Input: dimensioned drawing with shaded views. Units: mm. Origin: part minimum x, y, z. A direction names the side the tool comes from. Round coordinates to 2 decimals unless told otherwise and drop trailing zeros. Write each loop counter-clockwise with the first axis right and the second up, starting at its lowest first coordinate (ties: lowest second). Pieces come first, ordered by that corner, then holes. Notation, with made-up numbers: M -32,82.5 L -4,82.5 A9 ccw -4,92.5 Z; hole C 2.25,-34 d10. An arc over 180 degrees is marked long. Answer as CSV lines item,"result". Start each with the question number.
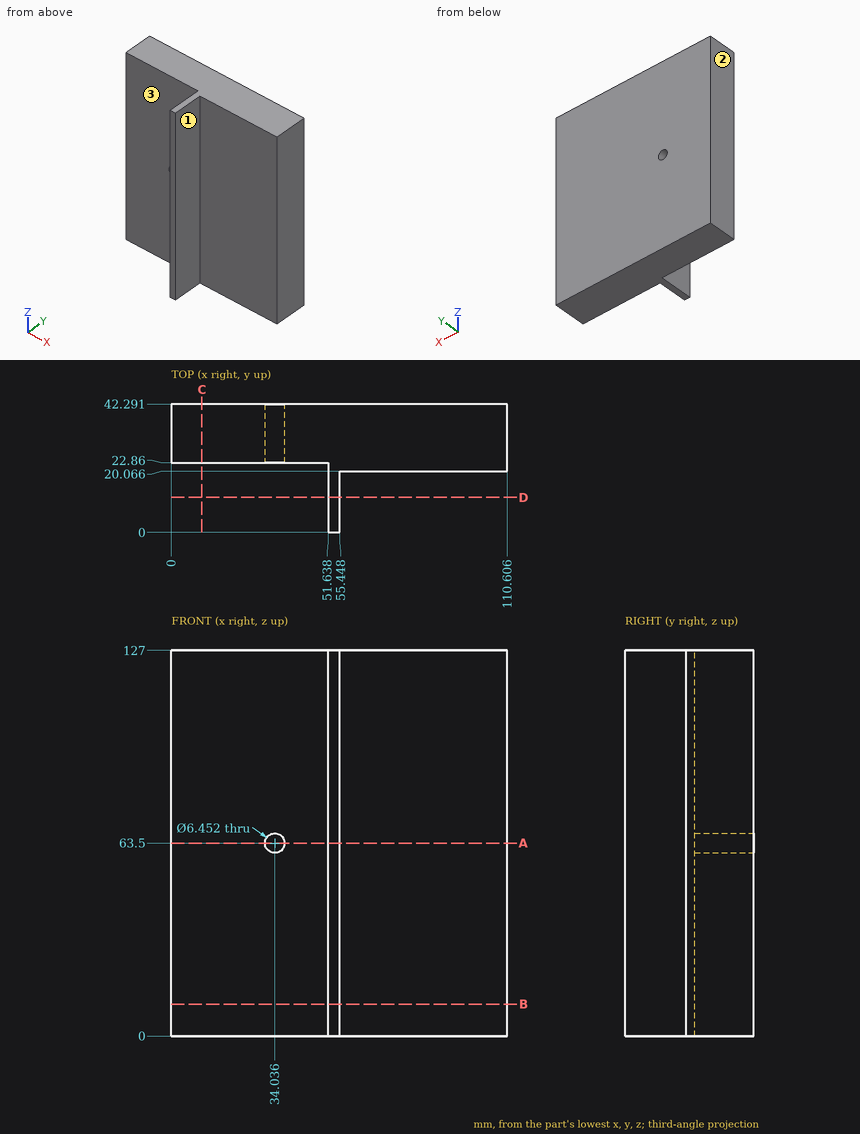
Item 1: Cut plane C-C, the plane x = 10. Return loops of the section in (y, z), plus the area to 3 significant figures.
Item 2: Cut plane D-D, the plane y = 11.5. Return loops of the section in (x, z).
Item 3: Cut plane B-B, the plane z = 10.5. Return loops of the section in (x, y).
Item 4: Cut plane A-A, the plane z = 63.5. Return loops of the section in (x, y), plus the area to 4 significant figures.
Item 5: Pin query (flat end, axial travel): pin 1 Ø1.5 at (x, z) = (22.5, 112) entering from -Y; pin 2 Ø5 at (x, z) = (34.036, 63.5) entering from +Y; pin 3 Ø16.5 at (x, z) = (86.5, 65) entering from -Y. Return the tip coordinate at first contact, or that it passes through.
Item 6: Access query for the marked faces 1, 2 and 3. Directions: +Z, -Z, +X, -X, +Y, -Y. A direction counts if a zero-diameter tool reaches every point of the face in a straight line with its end or side. Return the directions, or none.
Item 7: Line query: line 1 (Y direction, x = 48, z = 102.5); line 2 (X direction, y = 16, z = 29.5); line 3 (Y direction, x = 98, z = 79.5). Output: solid intervals per line, ascending. Write a range as [from, to].
Results list:
1,outline,"M 22.86,0 L 42.29,0 L 42.29,127 L 22.86,127 Z"
1,area,"2,470 mm²"
2,outline,"M 51.64,0 L 55.45,0 L 55.45,127 L 51.64,127 Z"
3,outline,"M 0,22.86 L 51.64,22.86 L 51.64,0 L 55.45,0 L 55.45,20.07 L 110.61,20.07 L 110.61,42.29 L 0,42.29 Z"
4,outline,"M 0,22.86 L 30.81,22.86 L 30.81,42.29 L 0,42.29 Z; M 37.26,22.86 L 51.64,22.86 L 51.64,0 L 55.45,0 L 55.45,20.07 L 110.61,20.07 L 110.61,42.29 L 37.26,42.29 Z"
4,area,"2,265 mm²"
5,pin 1,"y = 22.86"
5,pin 2,"through"
5,pin 3,"y = 20.07"
6,face 1,"+Z, -Z, +X, -Y"
6,face 2,"+Z, -Z, -X, +Y, -Y"
6,face 3,"+Z, -Z, -X, -Y"
7,line 1,"[22.86, 42.29]"
7,line 2,"[51.64, 55.45]"
7,line 3,"[20.07, 42.29]"
